from build123d import *

# Parameters (mm, degrees)
SKETCH_1_R      = 7
EXTRUDE_1_DEPTH = 16.25
EXTRUDE_START   = 2.5
SKETCH_2_R      = 8.5
EXTRUDE_2_DEPTH = 2


with BuildPart() as part:
    # 草图1 → 凸台-拉伸1 (new body, symmetric)
    with BuildSketch(Plane(origin=(0, 0, 0), x_dir=(1, 0, 0), z_dir=(0, 1, 0))):
        Circle(SKETCH_1_R)
    extrude(amount=EXTRUDE_1_DEPTH, both=True)

    # 草图2 → 凸台-拉伸2 (add)
    with BuildSketch(Plane(origin=(0, 0, 0), x_dir=(1, 0, 0), z_dir=(0, 1, 0)).offset(EXTRUDE_START)):
        Circle(SKETCH_2_R)
    extrude_2 = extrude(amount=EXTRUDE_2_DEPTH)

    # 镜向1: 凸台-拉伸2 across plane
    add(extrude_2.mirror(Plane.ZX))


solid = part.part
Geometry: final body of the model. Coordinates: model frame, mm. A direction names the side the tool comes from. Round coordinates to 2 decimals unless told otherwise and drop trailing zeros. Loops run counter-clockwise (first coordinate to the right, second up) from the corner with the lowest first, then second, coordinate; pieces in that order, holes last. Notation, with made-up numbers: M 5.25,80.25 L 64.25,80.25 A21 cw 64.25,118.25 Z; hole C -35,89.25 d6. An arc over 180 degrees is marked long. One line per question, with ' | ' between items.
(1) Cut plane C-C on y = -2. Return the cut outline in (x, z).
Check result:
outline: C 0,0 d14
(2) Pull-direction query (Y, two-part tool) for faces 1 (the flat face through (2, 2.5, -7)), 2 (the flat face through (0, 16.25, 0)), 3 (the cylindrical face through (4.57, 3.486, -7.167)); classes: +Y half, -Y half, draft (parallel to the pull), parting line (faces both ways), or undercut.
Check result:
face 1: undercut | face 2: +Y half | face 3: draft
(3) Cut plane A-A on x = 0. Return the cut outline in (y, z).
Check result:
outline: M -16.25,-7 L -4.5,-7 L -4.5,-8.5 L -2.5,-8.5 L -2.5,-7 L 2.5,-7 L 2.5,-8.5 L 4.5,-8.5 L 4.5,-7 L 16.25,-7 L 16.25,7 L 4.5,7 L 4.5,8.5 L 2.5,8.5 L 2.5,7 L -2.5,7 L -2.5,8.5 L -4.5,8.5 L -4.5,7 L -16.25,7 Z
(4) Material intervals for line 1 along Y through (x, z) = (6.25, 4.75); line 2 along Z through (x, y) = (-0.25, -15); line 3 along X through (y, z) = (12, -2), sorted ascending. Write a range as from..to.
Check result:
line 1: y = -4.5..-2.5, 2.5..4.5 | line 2: z = -7..7 | line 3: x = -6.71..6.71
(5) Contact query for flat-ended pins moving along their axis: P1, Ø1.5, axis at x = 3.5, y = -9, coming from the +Z side; P2, Ø3, axis at x = 4, y = 2.5, coming from the +Z side; P3, Ø8, axis at y = 3, z = 4.5, coming from the -X side. Output: stop coordinate, or through.
Check result:
P1: stops at z = 6.44 | P2: stops at z = 8.12 | P3: stops at x = -8.49
(6) Access query for faces 4 (the cylindrical face through (6.466, -10.293, 2.681)), 5 (the flat face through (2, -2.5, -7)), 6 (the cylindrical face through (4.57, -3.486, -7.167)), 7 (the cylindrical face through (6.466, 10.457, 2.681)). Directions: +Z, -Z, +X, -X, +Y, -Y. A direction counts if a zero-diameter tool reaches every point of the face in a straight line with its end or side. Return the directions, or none.
Check result:
face 4: -Y | face 5: none | face 6: +Y, -Y | face 7: +Y
(7) Cut plane B-B on z = 0. Return the cut outline in (x, y).
Check result:
outline: M -8.5,-4.5 L -7,-4.5 L -7,-16.25 L 7,-16.25 L 7,-4.5 L 8.5,-4.5 L 8.5,-2.5 L 7,-2.5 L 7,2.5 L 8.5,2.5 L 8.5,4.5 L 7,4.5 L 7,16.25 L -7,16.25 L -7,4.5 L -8.5,4.5 L -8.5,2.5 L -7,2.5 L -7,-2.5 L -8.5,-2.5 Z
